Read the model definition and answer for the solid it produces. Units are mm, in the model's axes. Face numbers are marked on the shaded views. A direction names the side the tool comes from. Coordinates: 2 decimals unless noted, no trailing zeros. Write each loop counter-clockwise with the first axis right and the second up, starting at its lowest first coordinate (ties: lowest second). Pieces come first, ordered by that corner, then holes. Notation, with made-up numbers: M 84,-13 L 124,-13 A38 ccw 124,25 Z; hole C 11.25,-31 d7. An arc over 180 degrees is marked long. Write item = value, one per line.
from build123d import *

# Parameters (mm, degrees)
SKETCH1_R           = 9.7
BOSS_EXTRUDE1_DEPTH = 20
CHAMFER1_SIZE       = 1.5


with BuildPart() as part:
    # Sketch1 → Boss-Extrude1 (new body)
    with BuildSketch(Plane(origin=(0, 0, 0), x_dir=(1, 0, 0), z_dir=(0, 1, 0))):
        with Locations(Location((0, 0, 0), (0, 0, 270))):
            Circle(SKETCH1_R)
        with BuildLine():
            Line((-1.45, -6), (1.45, -6))
            Line((1.45, -6), (1.45, -3.727935085))
            ThreePointArc((1.45, -3.727935085), (0, 4), (-1.45, -3.727935085))
            Line((-1.45, -3.727935085), (-1.45, -6))
        make_face(mode=Mode.SUBTRACT)
    extrude(amount=BOSS_EXTRUDE1_DEPTH)

    # Chamfer1
    chamfer1_edges = [part.edges().sort_by_distance(p)[0] for p in [
        (0, 20, -9.7),
    ]]
    chamfer(chamfer1_edges, length=CHAMFER1_SIZE)


solid = part.part
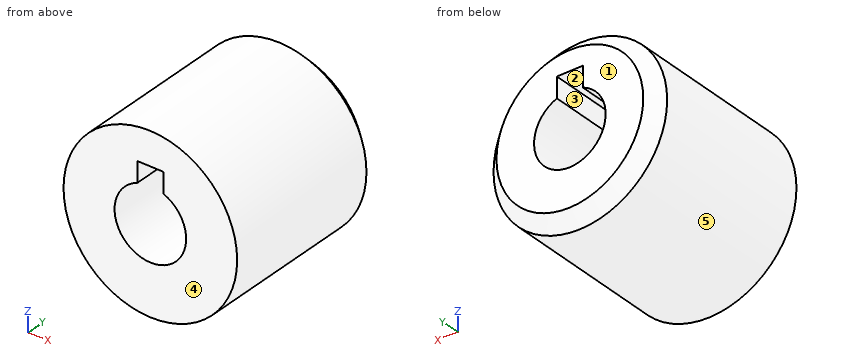
Item 1: Find section B-B (z = 0). Determine the outline of the cut face in (x, y), and give its area (3 significant figures).
Worked answers:
outline = M -9.7,0 L -4,0 L -4,20 L -8.2,20 L -9.7,18.5 Z; M 4,0 L 9.7,0 L 9.7,18.5 L 8.2,20 L 4,20 Z
area = 226 mm²
Item 2: Flat-ended cylindrical pins translate along their axes: pin 1 (2 mm diameter, centred on x = 6, y = 2, fed in from +Z); pin 2 (3 mm diameter, centred on x = -2.5, y = 13.5, fed in from -Z); pin 3 (3 mm diameter, centred on y = 7.5, z = 6.5, fed in from +X). Find the tip coordinate at first contact, or state that the pin passes through.
Worked answers:
pin_1 = 8.31
pin_2 = -9.65
pin_3 = 8.31
Item 3: Consider line 1 along X through (y, z) = (12.75, 0); line 2 along X through (y, z) = (6, -3.5); line 3 along Z through (x, y) = (2, 17.75). Determine where each line is inside the solid, lowest interval first. Write a range as from..to.
Worked answers:
line_1 = -9.7..-4, 4..9.7
line_2 = -9.05..-1.94, 1.94..9.05
line_3 = -9.49..-3.46, 3.46..9.49
Item 4: Find section A-A (x = 0). Determine the outline of the cut face in (y, z).
Worked answers:
outline = M 0,-9.7 L 18.5,-9.7 L 20,-8.2 L 20,-4 L 0,-4 Z; M 0,6 L 20,6 L 20,8.2 L 18.5,9.7 L 0,9.7 Z
Item 5: Find section C-C (y = 14.5). Determine the outline of the cut face in (x, z).
Worked answers:
outline = C 0,0 d19.4; hole M -1.45,3.73 A4 ccw long 1.45,3.73 L 1.45,6 L -1.45,6 Z
Item 6: Which of the six approach directions +Z, -Z, +X, -X, +Y, -Y give full straight-line access (tool end or side, diameter ignored) to the marked faces 1 and 2?
Worked answers:
face_1 = +Z, -Z, +X, -X, +Y
face_2 = +Y, -Y
Item 7: For a pull along X with two mould halves and no side action, classify the marked faces 3, 4 and 5 as released by +X, released by -X, zero draft, split by the parting line, or undercut.
Worked answers:
face_3 = undercut
face_4 = zero draft
face_5 = split by the parting line
